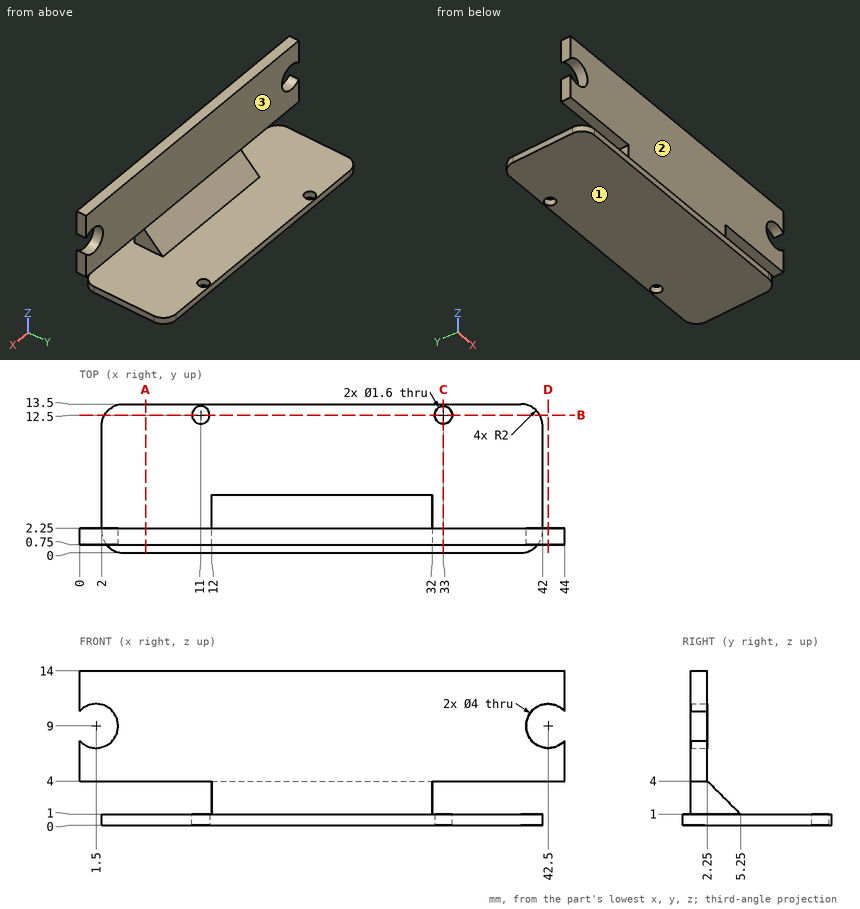
Input: dimensioned drawing with shaded views. Units: mm. Origin: part minimum x, y, z. A direction names the side the tool comes from. Give positions to 0.01 mm unless a question says otherwise; leave off trailing zeros. Order: outer loops, then holes, each group sorted by start corner. A loop starts at its lowest first (then second) coordinate and runs counter-clockwise, first axis right, second up. Notation, with made-up numbers: (-28.75, 10) -> (-2.75, 10) arc R15 cw to (-2.75, 39) -> close; hole circle Ø10 at (70, 62.5). An arc over 180 degrees is marked (long way). Write item = value, one per line.
Item 1: Ray query, probe 1 along Y at (x, z) = (11, 0.7); probe 2 along Z at (x, y) = (7, 1.25); probe 3 along Z at (x, y) = (42.5, 1.35). Return the intervals inside material, ascending.
Check result:
probe_1 = 0 to 11.7, 13.3 to 13.5
probe_2 = 0 to 1, 4 to 14
probe_3 = 4 to 7, 11 to 14
Item 2: Set-up query: the marked faces 1, 2 and 3. Return all of +Z, -Z, +X, -X, +Y, -Y with unobstructed straight access to the full face (end or side cutting, diameter ignored); none if empty.
Check result:
face_1 = -Z, +X, -X, +Y, -Y
face_2 = +Z, +X, -X, -Y
face_3 = +Z, +X, -X, +Y
Item 3: Section query A-A (x = 6). Output: boundary loops of the cut face in (y, z).
Check result:
outline = (0, 0) -> (13.5, 0) -> (13.5, 1) -> (0, 1) -> close; (0.75, 4) -> (2.25, 4) -> (2.25, 14) -> (0.75, 14) -> close
Item 4: Section query D-D (x = 42.5). Output: boundary loops of the cut face in (y, z), then the cut area to 3 significant figures.
Check result:
outline = (0.75, 4) -> (2.25, 4) -> (2.25, 7) -> (0.75, 7) -> close; (0.75, 11) -> (2.25, 11) -> (2.25, 14) -> (0.75, 14) -> close
area = 9.00 mm²
Item 5: Section query C-C (x = 33). Output: boundary loops of the cut face in (y, z), then the cut area to 3 significant figures.
Check result:
outline = (0, 0) -> (11.7, 0) -> (11.7, 1) -> (0, 1) -> close; (0.75, 4) -> (2.25, 4) -> (2.25, 14) -> (0.75, 14) -> close; (13.3, 0) -> (13.5, 0) -> (13.5, 1) -> (13.3, 1) -> close
area = 26.9 mm²
Item 6: Section query B-B (y = 12.5). Output: boundary loops of the cut face in (x, z), then the cut area to 3 significant figures.
Check result:
outline = (2.27, 0) -> (10.2, 0) -> (10.2, 1) -> (2.27, 1) -> close; (11.8, 0) -> (32.2, 0) -> (32.2, 1) -> (11.8, 1) -> close; (33.8, 0) -> (41.73, 0) -> (41.73, 1) -> (33.8, 1) -> close
area = 36.3 mm²
Item 7: Contact query for flat-ended pins moving along their axis: pin 1 (5 mm diameter, centred on x = 18, z = 7, fed in from +Y); pin 2 (1.5 mm diameter, centred on y = 4, z = 2.5, fed in from -X); pin 3 (5 mm diameter, centred on x = 28.5, z = 5, fed in from +Y). Output: stop coordinate, or through.
Check result:
pin_1 = 2.25
pin_2 = 12
pin_3 = 3.75
